Here's how the part is built. I have some questions about the finished solid (model axes, mm). A direction names the side the tool comes from. Give positions to 0.01 mm unless a question says otherwise; leave off trailing zeros. Loops run counter-clockwise (first coordinate to the right, second up) from the corner with the lowest first, then second, coordinate; pieces in that order, holes last.
Q1. I'm going to push flat-ended pins straight in: P1, Ø1, axis at x = 1, y = -1.5, coming from the +Z side; P2, Ø4, axis at x = 0, z = -4, coming from the +Y side; P3, Ø1.5, axis at y = -1, z = 2.5, coming from the +X side. Where does each tip first touch, or does it pass through?
Q2. For faces 4 (the face through (-1.32, 2.52, 1.93)), 5 (the face through (6, 0, 12.7)), which set-ups out of +Z, -Z, +X, -X, +Y, -Y let a thin tool reach every point of the face, with its end or its side?
Q3. Suppose I cut it at D-D (y = -2.5). List the corners of the cut face in (x, z) for me, and give its area (3 significant figures).
Q4. I need wall thicknesses on probe 1 along Z at (x, y) = (6.5, 0.25); probe 2 along Y at (x, z) = (6.5, -5); probe 3 along X at (y, z) = (0, -18.5) (3 decimals). Which ranges of each line are inside material? Lowest first, please.
Q5. Suppose I cut it at A-A (y = 0). List the corners of the cut face in (x, z) for me (3 decimals), and give its area (3 significant figures).
Q6. Thinking about a two-plate mould opening in Y: for faces 1 (the face through (6.29, 0.07, -37.59)), 2 (the face through (-6.35, 0, 0)), 3 (the face through (9.38, 0.95, -12.35)), which applies, pulls with the +Y half, pulls with the -Y half, needs draft (parallel to the pull), parting line crosses it, or undercut?
Q7. Suppose I cut it at B-B (z = 0). List the corners of the cut face in (x, y) for me (3 decimals), and give its area (3 significant figures).
Q8. Suppose I cut it at C-C (x = -3.25). List the corners of the cut face in (y, z) for me (3 decimals).
```python
from build123d import *

# Parameters (mm, degrees)
F0_W     = 12.7
F0_H     = 3.175
F2_R     = 3.175
F3_DEPTH = 3.175
F5_R     = 3.175
F6_DEPTH = 50.8
F7_R     = 10.16
F8_DEPTH = 25.4


with BuildPart() as f1:
    # F0 (on Top) → F1 (revolve)
    with BuildSketch(Plane.XY):
        with Locations((0, -1.5875)):
            Rectangle(F0_W, F0_H)
    revolve(axis=Axis((2.249268, 0, 0), (1, 0, 0)))

    # F2 (on Top) → F3 (cut, symmetric)
    with BuildSketch(Plane.XY):
        with Locations((6.35, 0)):
            Circle(F2_R)
    extrude(amount=F3_DEPTH, both=True, mode=Mode.SUBTRACT)

    # F5 (on offset) → F6 (join)
    with BuildSketch(Plane.XY.offset(12.7)):
        with Locations((6.35, 0)):
            Circle(F5_R)
    extrude(amount=-F6_DEPTH)

    # F7 (on Right) → F8 (cut)
    with BuildSketch(Plane.YZ):
        with Locations((0, -47.751164)):
            Circle(F7_R)
    extrude(amount=F8_DEPTH, mode=Mode.SUBTRACT)


solid = f1.part
```
Solutions:
1. P1: stops at z = 3.01
1. P2: stops at y = 2.47
1. P3: stops at x = 9.52
2. face 4: -X
2. face 5: +Z, +X, -X, +Y, -Y
3. outline: (-6.35, -1.96) - (4.39, -1.96) - (4.39, -37.9) - (8.31, -37.9) - (8.31, 12.7) - (4.39, 12.7) - (4.39, 1.96) - (-6.35, 1.96) - close
3. area: 240 mm2
4. probe 1: z = -37.59 to 12.7
4. probe 2: y = -3.17 to 3.17
4. probe 3: x = 3.175 to 9.525
5. outline: (-6.35, -3.175) - (3.175, -3.175) - (3.175, -37.591) - (9.525, -37.591) - (9.525, 12.7) - (3.175, 12.7) - (3.175, 3.175) - (-6.35, 3.175) - close
5. area: 380 mm2
6. face 1: undercut
6. face 2: needs draft
6. face 3: parting line crosses it
7. outline: (-6.35, -3.175) - (6.35, -3.175) arc R3.175 ccw to (6.35, 3.175) - (-6.35, 3.175) - close
7. area: 96.5 mm2
8. outline: circle Ø6.35 at (0, 0)
